from build123d import *

# Parameters (mm, degrees)
SKETCH022_W      = 131
SKETCH022_H      = 30
PAD007_DEPTH     = 10
SKETCH021_W      = 15
SKETCH021_H      = 30
PAD008_DEPTH     = 18.5
SKETCH023_W      = 25
SKETCH023_H      = 13.5
POCKET014_DEPTH  = 10
SKETCH020_R      = 3
POCKET015_DEPTH  = 10.001
SKETCH024_W      = 32.5
SKETCH024_H      = 30
POCKET016_DEPTH  = 5
SKETCH037_R      = 5
POCKET025_DEPTH  = 3
CHAMFER004_SIZE2 = 25
CHAMFER004_SIZE  = 10
CHAMFER005_SIZE  = 1


with BuildPart() as part:
    # Sketch022 → Pad007 (new body)
    with BuildSketch(Plane.XY):
        Rectangle(SKETCH022_W, SKETCH022_H)
    extrude(amount=PAD007_DEPTH)

    # Sketch021 (on Face5 of Pad007) → Pad008 (join)
    with BuildSketch(Plane(origin=(0, 0, 0), x_dir=(1, 0, 0), z_dir=(0, 0, -1))):
        with Locations((-58, 0)):
            Rectangle(SKETCH021_W, SKETCH021_H)
    extrude(amount=PAD008_DEPTH)

    # Sketch023 (on Face9 of Pad008) → Pocket014 (cut)
    with BuildSketch(Plane.YZ.offset(-50.5)):
        with Locations((2.5, -6.75)):
            Rectangle(SKETCH023_W, SKETCH023_H)
    extrude(amount=-POCKET014_DEPTH, mode=Mode.SUBTRACT)

    # Sketch020 (on Face5 of Pocket014) → Pocket015 (cut, through all)
    with BuildSketch(Plane(origin=(0, 0, 0), x_dir=(1, 0, 0), z_dir=(0, 0, -1))):
        with Locations((50.5, 0)):
            Circle(SKETCH020_R)
    extrude(amount=-POCKET015_DEPTH, mode=Mode.SUBTRACT)

    # Sketch024 → Pocket016 (cut)
    with BuildSketch(Plane.XY.offset(10)):
        with Locations((49.25, 0)):
            Rectangle(SKETCH024_W, SKETCH024_H)
    extrude(amount=-POCKET016_DEPTH, mode=Mode.SUBTRACT)

    # Sketch037 (on Face4 of Pocket016) → Pocket025 (cut)
    with BuildSketch(Plane(origin=(0, 0, 0), x_dir=(1, 0, 0), z_dir=(0, 0, -1))):
        with Locations((50.5, 0)):
            Circle(SKETCH037_R)
    extrude(amount=-POCKET025_DEPTH, mode=Mode.SUBTRACT)

    # Chamfer004
    chamfer004_edges = [part.edges().sort_by_distance(p)[0] for p in [
        (-50.5, 15, -16),
    ]]
    chamfer004_side = part.faces().sort_by_distance((-55.5, 15, -13.73817))[0]
    chamfer(chamfer004_edges, length=CHAMFER004_SIZE, length2=CHAMFER004_SIZE2, reference=chamfer004_side)

    # Chamfer005
    chamfer005_edges = [part.edges().sort_by_distance(p)[0] for p in [
        (-55.5, 2.5, -18.5),
        (-55.5, 2.5, -13.5),
        (-50.5, -12.5, -18.5),
        (-58, -15, -18.5),
        (-50.5, -15, -9.25),
        (-65.5, 0, -18.5),
        (-65.5, 15, -9.25),
        (-65.5, 15, 5),
        (-65.5, 0, 10),
        (-65.5, -15, 5),
        (-65.5, -15, -9.25),
    ]]
    chamfer(chamfer005_edges, length=CHAMFER005_SIZE)


solid = part.part
Geometry: final body of the model. Coordinates: model frame, mm. A direction names the side the tool comes from. Give positions to 0.01 mm unless a question says otherwise; leave off trailing zeros. Order: outer loops, then holes, each group sorted by start corner. A loop starts at its lowest first (then second) coordinate and runs counter-clockwise, first axis right, second up. Notation, with made-up numbers: (67, -16) -> (87, -16) arc R20 ccw to (87, 1) -> close; hole circle Ø8 at (40.5, -13). An arc over 180 degrees is marked (long way). Write each question's results on one line, items separated by ' | '.
1) Cut plane C-C (y = 0). Output: boundary loops of the cut face in (x, z).
Geometry says:
outline: (-65.5, -17.5) -> (-64.5, -18.5) -> (-55.58, -18.5) -> (-54.5, -17.5) -> (-54.5, -14.5) -> (-55.58, -13.5) -> (-60.5, -13.5) -> (-60.5, 0) -> (45.5, 0) -> (45.5, 3) -> (47.5, 3) -> (47.5, 5) -> (33, 5) -> (33, 10) -> (-64.5, 10) -> (-65.5, 9) -> close; (53.5, 3) -> (55.5, 3) -> (55.5, 0) -> (65.5, 0) -> (65.5, 5) -> (53.5, 5) -> close
2) Line query: line 1 along Y through (x, z) = (50.5, 4.3); line 2 along Y through (x, z) = (50.5, 1.9); line 3 along X through (y, z) = (0, 0.95). Output: solid intervals per line, ascending.
Geometry says:
line 1: y = -15 to -3, 3 to 15 | line 2: y = -15 to -5, 5 to 15 | line 3: x = -65.5 to 45.5, 55.5 to 65.5
3) First-contact query: pin 1 Ø2 at (y, z) = (-11.5, -9.5) entering from +X; pin 2 Ø2 at (x, y) = (40.5, -2) entering from -Z; pin 3 Ø2.5 at (y, z) = (7, 7) entering from +X. Flat tips, straight axial feed; report the tip coordinate or a pass-through.
Geometry says:
pin 1: stops at x = -50.5 | pin 2: stops at z = 0 | pin 3: stops at x = 33
4) Cut plane A-A (x = 50.5). Output: boundary loops of the cut face in (y, z), and give its area (3 significant figures).
Geometry says:
outline: (-15, 0) -> (-5, 0) -> (-5, 3) -> (-3, 3) -> (-3, 5) -> (-15, 5) -> close; (3, 3) -> (5, 3) -> (5, 0) -> (15, 0) -> (15, 5) -> (3, 5) -> close | area: 108 mm²
5) Set-up query: faces 5 (the face through (-58, -4, -13.5)), 6 (the face through (-50.5, -12, -9)), 7 (the face through (53, 2, 3)), 8 (the face through (-55.43, 2.33, -15.98)), 9 (the face through (33, 0, 8)). Return all of +Z, -Z, +X, -X, +Y, -Y with unobstructed straight access to the full face (end or side cutting, diameter ignored); none if empty.
Geometry says:
face 5: +X, +Y | face 6: -Z, +X, +Y, -Y | face 7: -Z | face 8: -Z, +X, +Y | face 9: +Z, +X, +Y, -Y
6) Cut plane B-B (z = -10.5). Output: boundary loops of the cut face in (x, y), and give its area (4 significant figures).
Geometry says:
outline: (-65.5, -14) -> (-64.5, -15) -> (-51.5, -15) -> (-50.5, -14) -> (-50.5, -10) -> (-60.5, -10) -> (-60.5, 15) -> (-64.5, 15) -> (-65.5, 14) -> close | area: 198.5 mm²
7) Cut plane D-D (y = 9). Output: boundary loops of the cut face in (x, z), and give its area (3 significant figures).
Geometry says:
outline: (-65.5, -17.5) -> (-64.5, -18.5) -> (-59.18, -18.5) -> (-58.1, -17.5) -> (-58.1, -14.5) -> (-59.18, -13.5) -> (-60.5, -13.5) -> (-60.5, 0) -> (65.5, 0) -> (65.5, 5) -> (33, 5) -> (33, 10) -> (-64.5, 10) -> (-65.5, 9) -> close | area: 1,250 mm²
8) Draft query along X for faces 1 (the face through (65.5, 0, 2)), 2 (the face through (-65.5, 0, -4)), 3 (the face through (2, 0, 0)), 4 (the face through (47.5, -0.1, 4)). Return one class per face: released by +X, released by -X, zero draft, split by the parting line, or undercut.
Geometry says:
face 1: released by +X | face 2: released by -X | face 3: zero draft | face 4: undercut
